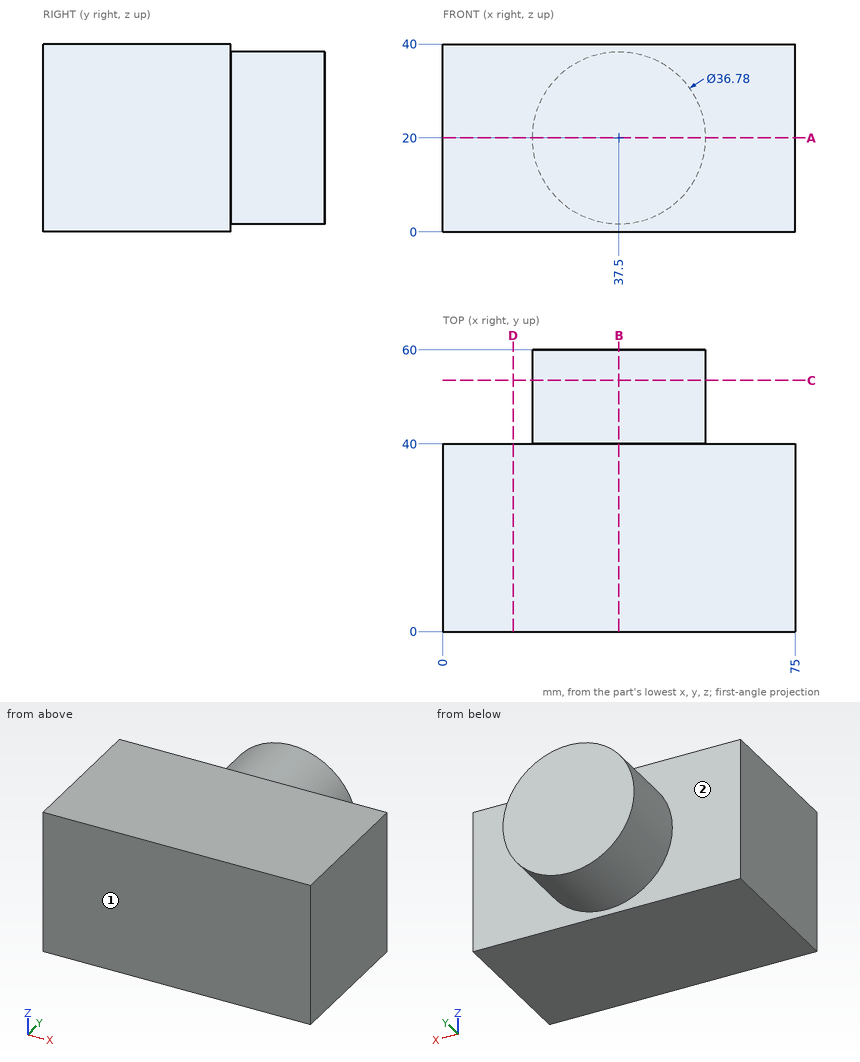
The drawing under review shows one solid part. Ordinate dimensions are in mm from its lowest x, y, z. A direction names the side the tool comes from. Round coordinates to 2 decimals unless told otherwise and drop trailing zeros. Order: outer loops, then holes, each group sorted by start corner. A loop starts at its lowest first (then second) coordinate and runs counter-clockwise, first axis right, second up. Notation, with made-up numbers: M -8,86 L -1,86 A23 cw -1,103 Z; hole C 18,-32.5 d5. An arc over 180 degrees is marked long. Answer as CSV lines item,"result". Start each with the question number.
1) For pin 1 Ø5 at (x, z) = (8.5, 15) entering from +Y; pin 2 Ø1 at (y, z) = (42.5, 24) entering from -X; pin 3 Ø3 at (x, y) = (48, 46) entering from +Z, all flat-tipped, find the tip position at first contact; note any pin that passes through.
2) Add section B-B (x = 37.5). Give the boundary of the cut face in (y, z).
3) Add section C-C (y = 53.5). Give the boundary of the cut face in (x, z).
4) Tool access review of the marked faces 1 and 2: name each direction out of +Z, -Z, +X, -X, +Y, -Y from which nothing blocks a thin tool from reaching the whole face with its end or side.
5) Add section D-D (x = 15). Give the boundary of the cut face in (y, z).
6) Wall thickness on line 1 along Y through (x, z) = (64, 36); line 2 along X through (y, z) = (43, 19); line 3 along X through (y, z) = (43, 32): over which ranges is each line inside the solid? List them lowest first. Write a range as [from, to].
7) Add section A-A (z = 20). Give the boundary of the cut face in (x, y), then the cut area to 3 significant figures.
Resolved:
1,pin 1,"y = 40"
1,pin 2,"x = 19.45"
1,pin 3,"z = 36.04"
2,outline,"M 0,0 L 40,0 L 40,1.61 L 60,1.61 L 60,38.39 L 40,38.39 L 40,40 L 0,40 Z"
3,outline,"C 37.5,20 d36.78"
4,face 1,"+Z, -Z, +X, -X, -Y"
4,face 2,"+Y"
5,outline,"M 0,0 L 40,0 L 40,40 L 0,40 Z"
6,line 1,"[0, 40]"
6,line 2,"[19.14, 55.86]"
6,line 3,"[23.56, 51.44]"
7,outline,"M 0,0 L 75,0 L 75,40 L 55.89,40 L 55.89,60 L 19.11,60 L 19.11,40 L 0,40 Z"
7,area,"3,740 mm^2"
